```python
from build123d import *

# Parameters (mm, degrees)
SKETCH_1_R      = 2.475
EXTRUDE_1_DEPTH = 10
FILLET_1_R      = 2


with BuildPart() as part:
    # Эскиз1 → Бобышка-Вытянуть1 (new body)
    with BuildSketch(Plane(origin=(0, 0, 0), x_dir=(1, 0, 0), z_dir=(0, 1, 0))):
        with BuildLine():
            Line((-7.5, 66), (-7.5, 55.400571017))
            ThreePointArc((-7.5, 55.400571017), (-10.276982955, 37.358223046), (-18.350877343, 20.985984836))
            Line((-18.350877343, 20.985984836), (-30.23406431, 4.015035054))
            ThreePointArc((-30.23406431, 4.015035054), (-30.709075832, -3.232240293), (-24.5, -7))
            Line((-24.5, -7), (24.5, -7))
            ThreePointArc((24.5, -7), (30.709075832, -3.232240293), (30.23406431, 4.015035054))
            Line((30.23406431, 4.015035054), (18.350877343, 20.985984836))
            ThreePointArc((18.350877343, 20.985984836), (10.276982955, 37.358223046), (7.5, 55.400571017))
            Line((7.5, 55.400571017), (7.5, 66))
            ThreePointArc((7.5, 66), (0, 73.5), (-7.5, 66))
        make_face()
        with Locations(Location((-24.5, 0, 0), (0, 0, 270))):
            Circle(SKETCH_1_R, mode=Mode.SUBTRACT)
        with Locations(Location((24.5, 0, 0), (0, 0, 270))):
            Circle(SKETCH_1_R, mode=Mode.SUBTRACT)
        with BuildLine():
            Line((10.1593569, 15.250220472), (18.737053619, 3))
            Line((18.737053619, 3), (-18.737053619, 3))
            Line((-18.737053619, 3), (-10.1593569, 15.250220472))
            ThreePointArc((-10.1593569, 15.250220472), (-4.1514168, 25.618747591), (0, 36.860074799))
            ThreePointArc((0, 36.860074799), (4.1514168, 25.618747591), (10.1593569, 15.250220472))
        make_face(mode=Mode.SUBTRACT)
    extrude(amount=EXTRUDE_1_DEPTH)

    # Скругление1
    fillet_1_edges = [part.edges().sort_by_distance(p)[0] for p in [
        (0, 5, -36.860074799),
        (-18.737053619, 5, -3),
        (18.737053619, 5, -3),
    ]]
    fillet(fillet_1_edges, radius=FILLET_1_R)


solid = part.part
```
For this review, take the finished solid that the model builds, in its own axes (mm). A direction names the side the tool comes from. Coordinates: 2 decimals unless noted, no trailing zeros. Write each loop counter-clockwise with the first axis right and the second up, starting at its lowest first coordinate (ties: lowest second). Pieces come first, ordered by that corner, then holes. Notation, with made-up numbers: (50.25, -38.75) -> (99.25, -38.75) arc R17 ccw to (99.25, -9.75) -> close; hole circle Ø1 at (-15.5, 56). An arc over 180 degrees is marked (long way). Put each result on its own line as item: value.
Q1. Wall thickness on L1, parallel to X at y = 2.5, z = 0 (3 decimals); L2, parallel to X at y = 4.25, z = 1; L3, parallel to X at y = 4.75, z = -59: over which ranges is each line inside the solid? List them lowest first.
From the geometry:
L1: x = -31.5 to -26.975, -22.025 to 22.025, 26.975 to 31.5
L2: x = -31.43 to -26.76, -22.24 to 22.24, 26.76 to 31.43
L3: x = -7.5 to 7.5
Q2. Take a section at D-D, the plane z = -57.5. State the section outline as (x, y) points, then the cut area to 3 significant figures.
From the geometry:
outline: (-7.5, 0) -> (7.5, 0) -> (7.5, 10) -> (-7.5, 10) -> close
area: 150 mm2
Q3. Clearance check with flat-ended pins moving along their axes: pin 1 Ø2 at (y, z) = (6.5, -21.5) entering from -X; pin 2 Ø1.5 at (y, z) = (3, -22.5) entering from +X; pin 3 Ø4 at (x, z) = (8.5, -52) entering from -Y; pin 4 Ø1 at (y, z) = (5, -9) entering from +X. State where each tip first meets the part, or that it passes through.
From the geometry:
pin 1: stops at x = -18.69
pin 2: stops at x = 17.82
pin 3: stops at y = 0
pin 4: stops at x = 27.09
Q4. Tool access review of faces 1 (the cylindrical face through (0.16, 4.93, -73.5)), 2 (the flat face through (-7.5, 5, -61)), 3 (the cylindrical face through (16.655, 5.07, -4.05)): name each direction out of +Z, -Z, +X, -X, +Y, -Y from which nothing blocks a thin tool from reaching the whole face with its end or side.
From the geometry:
face 1: -Z, +Y, -Y
face 2: -Z, -X, +Y, -Y
face 3: +Y, -Y
Q5. Take a section at A-A, the plane z = 0. State the section outline as (x, y) points (3 decimals), then the cut area to 3 significant figures.
From the geometry:
outline: (-31.5, 0) -> (-26.975, 0) -> (-26.975, 10) -> (-31.5, 10) -> close; (-22.025, 0) -> (22.025, 0) -> (22.025, 10) -> (-22.025, 10) -> close; (26.975, 0) -> (31.5, 0) -> (31.5, 10) -> (26.975, 10) -> close
area: 531 mm2
Q6. Take a section at B-B, the plane z = -29.5. State the section outline as (x, y) points.
From the geometry:
outline: (-13.38, 0) -> (-2.47, 0) -> (-2.47, 10) -> (-13.38, 10) -> close; (2.47, 0) -> (13.38, 0) -> (13.38, 10) -> (2.47, 10) -> close
Q7. The part is to be moulded in two halves that separate along Z. For faces 4 (the cylindrical face through (30.659, 4.93, 3.327)), 5 (the cylindrical face through (5.454, 4.93, -22.992)), 6 (the cylindrical face through (10.355, 4.93, -37.114)), say which applies: +Z half, -Z half, draft (parallel to the pull), parting line (faces both ways), or undercut.
From the geometry:
face 4: parting line
face 5: undercut
face 6: -Z half
Q8. Take a section at C-C, the plane y = 3. Count the separate pieces of the cut face and the enclosed holes in it, then the cut area to 3 significant figures.
From the geometry:
separate pieces: 1
enclosed holes: 3
area: 1,930 mm2
